from build123d import *

# Parameters (mm, degrees)
STOCK_DEPTH                                      = 114.3
CBORE_FOR_1_4_SOCKET_HEAD_CAP_SCREW1_D           = 6.7564
CBORE_FOR_1_4_SOCKET_HEAD_CAP_SCREW1_CBORE_D     = 11.1125
CBORE_FOR_1_4_SOCKET_HEAD_CAP_SCREW1_CBORE_DEPTH = 6.35
CHAMFER1_SIZE                                    = 1.5875


with BuildPart() as part:
    # Sketch1 → stock (new body)
    with BuildSketch(Plane.XY):
        with BuildLine():
            Line((7.777129933, -1.5875), (17.937129933, -1.5875))
            Line((17.937129933, -1.5875), (17.937129933, -14.2875))
            Line((17.937129933, -14.2875), (-17.937129933, -14.2875))
            Line((-17.937129933, -14.2875), (-17.937129933, -1.5875))
            Line((-17.937129933, -1.5875), (-7.777129933, -1.5875))
            ThreePointArc((-7.777129933, -1.5875), (0, -7.9375), (7.777129933, -1.5875))
        make_face()
    extrude(amount=STOCK_DEPTH)

    # CBORE for 1/4 Socket Head Cap Screw1 (through all)
    with Locations(Plane(origin=(0, -14.2875, 0), x_dir=(-1, 0, 0), z_dir=(0, -1, 0))):
        with Locations((12.7, -19.05), (12.7, -57.15), (12.7, -95.25), (-12.7, -95.25), (-12.7, -57.15), (-12.7, -19.05)):
            CounterBoreHole(CBORE_FOR_1_4_SOCKET_HEAD_CAP_SCREW1_D / 2, CBORE_FOR_1_4_SOCKET_HEAD_CAP_SCREW1_CBORE_D / 2, CBORE_FOR_1_4_SOCKET_HEAD_CAP_SCREW1_CBORE_DEPTH)

    # Chamfer1
    chamfer1_edges = [part.edges().sort_by_distance(p)[0] for p in [
        (17.937129933, -14.2875, 105.702952602),
        (-17.937129933, -14.2875, 105.702952602),
        (17.937129933, -14.2875, 8.597047398),
        (7.14375, -14.2875, 19.05),
        (17.937129933, -14.2875, 38.1),
        (7.14375, -14.2875, 57.15),
        (0, -14.2875, 114.3),
        (17.937129933, -14.2875, 76.2),
        (7.14375, -14.2875, 95.25),
        (-17.937129933, -14.2875, 76.2),
        (-7.14375, -14.2875, 95.25),
        (-17.937129933, -14.2875, 38.1),
        (-7.14375, -14.2875, 57.15),
        (0, -14.2875, 0),
        (-17.937129933, -14.2875, 8.597047398),
        (-7.14375, -14.2875, 19.05),
    ]]
    chamfer(chamfer1_edges, length=CHAMFER1_SIZE)


solid = part.part
Model file for the job. Use its own axes, mm. A direction names the side the tool comes from. Give positions to 0.01 mm unless a question says otherwise; leave off trailing zeros. Loops run counter-clockwise (first coordinate to the right, second up) from the corner with the lowest first, then second, coordinate; pieces in that order, holes last.
1) Pull direction Z, two halves, no side cores. Call faces 1 (the flat face through (-16.3, -1.588, 56.3)), 2 (the flat face through (0.3, -8.3, 114.3)), 3 (the cylindrical face through (7.15, -10.35, 57.37)): +Z half, -Z half, draft (parallel to the pull), parting line (faces both ways), or undercut.
2) Saw through at B-B (y = -3.5). Write the cut outline in (x, z).
3) Saw through at C-C (y = -9.5). Write the cut outline in (x, z).
4) Tool access for faces 4 (the flat face through (10, -7.938, 60)), 5 (the flat face through (-17.937, -7, 56)): list every direction of +Z, -Z, +X, -X, +Y, -Y with a clear straight run to the whole face (end or side of a thin tool).
5) Wall check: line 1 (Z direction, x = -12.7, y = -10.35); line 2 (Z direction, x = 12.7, y = -6.5); line 3 (X direction, y = -6.5, z = 95.25). Give the ranges that are in metal, low to high.
6) Saw through at A-A (z = 19.05). Write the cut outline in (x, y) (1 decimal), plus the area to 3 significant figures.
7) Flat gauge pins, fed straight in: pin 1 Ø12 at (x, z) = (-11, 17) entering from -Y; pin 2 Ø9 at (x, z) = (12.7, 19.05) entering from -Y; pin 3 Ø8.5 at (x, z) = (11.5, 56.5) entering from -Y; pin 4 Ø8.5 at (x, z) = (-15, 55.5) entering from -Y. Where does each tip first touch, or does it go through?
8) Saw through at D-D (x = 0). Write the cut outline in (y, z), plus the area to 3 significant figures.
Answer block:
1. face 1: draft
1. face 2: +Z half
1. face 3: undercut
2. outline: (-17.94, 0) - (-7.12, 0) - (-7.12, 114.3) - (-17.94, 114.3) - close; (7.12, 0) - (17.94, 0) - (17.94, 114.3) - (7.12, 114.3) - close; hole circle Ø6.76 at (-12.7, 19.05); hole circle Ø6.76 at (-12.7, 57.15); hole circle Ø6.76 at (-12.7, 95.25); hole circle Ø6.76 at (12.7, 19.05); hole circle Ø6.76 at (12.7, 57.15); hole circle Ø6.76 at (12.7, 95.25)
3. outline: (-17.94, 0) - (17.94, 0) - (17.94, 17.19) arc R5.56 cw (long way) to (17.94, 20.91) - (17.94, 55.29) arc R5.56 cw (long way) to (17.94, 59.01) - (17.94, 93.39) arc R5.56 cw (long way) to (17.94, 97.11) - (17.94, 114.3) - (-17.94, 114.3) - (-17.94, 97.11) arc R5.56 cw (long way) to (-17.94, 93.39) - (-17.94, 59.01) arc R5.56 cw (long way) to (-17.94, 55.29) - (-17.94, 20.91) arc R5.56 cw (long way) to (-17.94, 17.19) - close
4. face 4: -Y
4. face 5: +Z, -Z, -X, +Y, -Y
5. line 1: z = 0 to 13.49, 24.61 to 51.59, 62.71 to 89.69, 100.81 to 114.3
5. line 2: z = 0 to 15.67, 22.43 to 53.77, 60.53 to 91.87, 98.63 to 114.3
5. line 3: x = -17.94 to -16.08, -9.32 to -4.56, 4.56 to 9.32, 16.08 to 17.94
6. outline: (-17.9, -7.9) - (-16.1, -7.9) - (-16.1, -1.6) - (-17.9, -1.6) - close; (-9.3, -7.9) - (-7.1, -7.9) - (-7.1, -12.7) - (-5.6, -14.3) - (5.6, -14.3) - (7.1, -12.7) - (7.1, -7.9) - (9.3, -7.9) - (9.3, -1.6) - (7.8, -1.6) arc R7.9 cw to (-7.8, -1.6) - (-9.3, -1.6) - close; (16.1, -7.9) - (17.9, -7.9) - (17.9, -1.6) - (16.1, -1.6) - close
6. area: 156 mm2
7. pin 1: stops at y = -14.29
7. pin 2: stops at y = -7.94
7. pin 3: stops at y = -12.76
7. pin 4: stops at y = -13.97
8. outline: (-14.29, 1.59) - (-12.7, 0) - (-7.94, 0) - (-7.94, 114.3) - (-12.7, 114.3) - (-14.29, 112.71) - close
8. area: 723 mm2
